```python
from build123d import *

# Parameters (mm, degrees)
F0_R     = 10.079521
F1_DEPTH = 25.4
F2_R     = 6.132102
F3_T     = -2.54


with BuildPart() as f1:
    # F0 (on Front) → F1 (new body)
    with BuildSketch(Plane.XZ):
        Circle(F0_R)
    extrude(amount=F1_DEPTH)

    # F2
    f2_edges = [f1.edges().sort_by_distance(p)[0] for p in [
        (-10.079521, -25.4, 0),
    ]]
    fillet(f2_edges, radius=F2_R)

    # F3
    f3_openings = [f1.faces().sort_by_distance(p)[0] for p in [
        (0, 0, 0),
    ]]
    offset(amount=F3_T, openings=f3_openings)


solid = f1.part
```
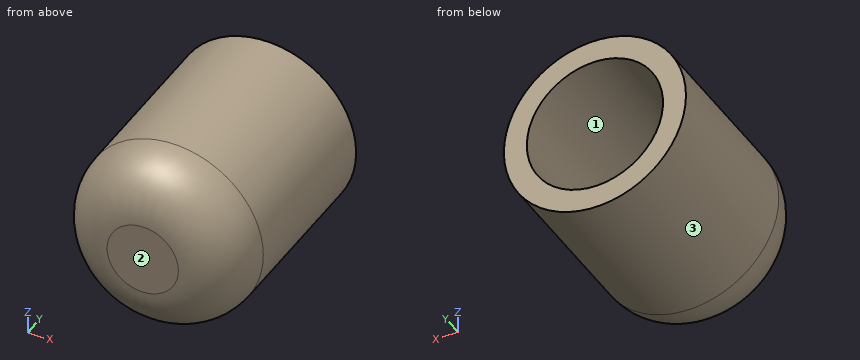
Verification items for the finished model (mm, model axes). Face numbers are marked on the shaded views. Round coordinates to 2 decimals unless told otherwise and drop trailing zeros. Loops run counter-clockwise (first coordinate to the right, second up) from the corner with the lowest first, then second, coordinate; pieces in that order, holes last. Notation, with made-up numbers: (86.5, 4.25) -> (111.5, 4.25) arc R33 ccw to (111.5, 32.25) -> close; hole circle Ø11 at (-13, 74.5). An arc over 180 degrees is marked (long way). Answer as a JSON object with one key per item and string values.
Q1. Section check A-A (y = -15). Record the boundary of the cut face in (x, z), then the cut area to 3 significant figures.
Data:
{"outline": "circle Ø20.16 at (0, 0); hole circle Ø15.08 at (0, 0)", "area": "141 mm2"}
Q2. Scan lines: line 1 (Z direction, x = 0, y = -5.75); line 2 (Y direction, x = 1.25, z = 2.75); line 3 (X direction, y = -21.25, z = -5.5). Record each from-to range of solid material in increasing order. Write a range as from..to.
Data:
{"line 1": "z = -10.08..-7.54, 7.54..10.08", "line 2": "y = -25.4..-22.86", "line 3": "x = -8.05..-4.24, 4.24..8.05"}
Q3. Draft check along Z on the marked faces 1, 2 and 3. Enter one of: pulls with the +Z half, pulls with the -Z half, needs draft (parallel to the pull), parting line crosses it, or undercut.
Data:
{"face 1": "undercut", "face 2": "needs draft", "face 3": "parting line crosses it"}
Q4. Go/stop test with flat-tipped pins: P1, Ø8, axis at x = 4.5, y = -18.5, coming from the -Z side; P2, Ø4, axis at x = 0, z = 1, coming from the +Y side; P3, Ø1.5, axis at y = -15, z = 1, coming from the +X side. Record where each tip stops, or that it passes through.
Data:
{"P1": "stops at z = -10.07", "P2": "stops at y = -22.86", "P3": "stops at x = 10.08"}
